Can you work these out from the model? Positions are in its coordinate system, mm. Round coordinates to 2 decimals unless told otherwise and drop trailing zeros. Order: outer loops, then holes, each group sorted by start corner. A loop starts at its lowest first (then second) coordinate and runs counter-clockwise, first axis right, second up. Notation, with made-up numbers: M 6,51 L 25,51 A19 cw 25,58 Z; hole C 40,65.25 d11. An arc over 180 degrees is marked long. One line per question, with ' | ' between items.
```python
from build123d import *

# Parameters (mm, degrees)
F1_DEPTH = 1460
F3_D     = 5.5
F3_DEPTH = 14.4
F3_TIP   = 1.6523667023
F5_DEPTH = 50.001


# Not quite as in the source:
# - a feature names something its author has since deleted; it is built from what else it names


with BuildPart() as f1:
    # F0 (on Front) → F1 (new body)
    with BuildSketch(Plane.XZ):
        with BuildLine():
            Line((-20, -50), (20, -50))
            ThreePointArc((20, -50), (23.5355339059, -48.5355339059), (25, -45))
            Line((25, -45), (25, 45))
            ThreePointArc((25, 45), (23.5355339059, 48.5355339059), (20, 50))
            Line((20, 50), (-20, 50))
            ThreePointArc((-20, 50), (-23.5355339059, 48.5355339059), (-25, 45))
            Line((-25, 45), (-25, -45))
            ThreePointArc((-25, -45), (-23.5355339059, -48.5355339059), (-20, -50))
        make_face()
        with BuildLine():
            ThreePointArc((-17.5, -45), (-19.267766953, -44.267766953), (-20, -42.5))
            Line((-20, -42.5), (-20, 42.5))
            ThreePointArc((-20, 42.5), (-19.267766953, 44.267766953), (-17.5, 45))
            Line((-17.5, 45), (17.5, 45))
            ThreePointArc((17.5, 45), (19.267766953, 44.267766953), (20, 42.5))
            Line((20, 42.5), (20, -42.5))
            ThreePointArc((20, -42.5), (19.267766953, -44.267766953), (17.5, -45))
            Line((17.5, -45), (-17.5, -45))
        make_face(mode=Mode.SUBTRACT)
    extrude(amount=-F1_DEPTH)

    # F3
    with Locations(Plane.XY.offset(50)):
        with Locations((0, 50), (0, 250), (0, 450), (0, 650), (0, 850), (0, 1050), (0, 1250), (0, 1450)):
            Hole(F3_D / 2, depth=F3_DEPTH)
            with Locations((0, 0, -(F3_DEPTH + F3_TIP / 2))):  # 118° drill point
                Cone(0, F3_D / 2, F3_TIP, mode=Mode.SUBTRACT)

    # F4 (on face) → F5 (cut, through all)
    with BuildSketch(Plane.YZ.offset(25)):
        with BuildLine():
            Line((1450.4894832185, 29.8696045958), (1450.4894832185, 35.6303954042))
            ThreePointArc((1450.4894832185, 35.6303954042), (1444.1498086534, 42.4982734143), (1437.5003786468, 35.9298411402))
            Line((1437.5003786468, 35.9298411402), (1437.5003786468, 29.5701588598))
            ThreePointArc((1437.5003786468, 29.5701588598), (1444.1498086534, 23.0017265857), (1450.4894832185, 29.8696045958))
        make_face()
        with BuildLine():
            Line((1437.5008297564, -29.6038563662), (1437.5000000547, -35.999156715))
            ThreePointArc((1437.5000000547, -35.999156715), (1444.0002415297, -42.4999999955), (1450.4999998647, -35.9986736556))
            Line((1450.4999998647, -35.9986736556), (1450.4987003133, -29.6299778371))
            ThreePointArc((1450.4987003133, -29.6299778371), (1444.0130628488, -23.000013126), (1437.5008297564, -29.6038563662))
        make_face()
    extrude(amount=-F5_DEPTH, mode=Mode.SUBTRACT)


solid = f1.part
```
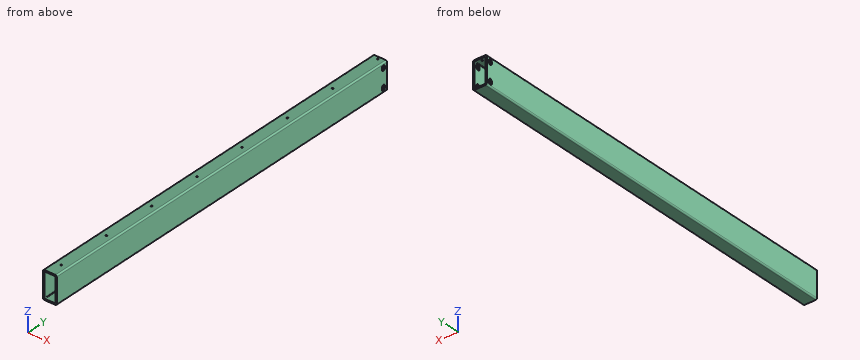
(1) Please list where these lines run through material, in increasing order: probe 1 along Z at (x, y) = (-14.5, 572); probe 2 along X at (y, z) = (526, -38); probe 3 along Z at (x, y) = (18.5, 610.5). Write a range as [from, to].
Final values:
probe 1: [-50, -45], [45, 50] | probe 2: [-25, -20], [20, 25] | probe 3: [-50, -44.79], [44.79, 50]
(2) If we section it at A-A on z = -6: Please give me the cut outline in (x, y), plus the area to 3 significant figures.
Final values:
outline: M -25,0 L -20,0 L -20,1460 L -25,1460 Z; M 20,0 L 25,0 L 25,1460 L 20,1460 Z | area: 14,600 mm^2
(3) If we section it at B-B on y = 1032.5: Please give me the cut outline in (x, z).
Final values:
outline: M -25,-45 A5 ccw -20,-50 L 20,-50 A5 ccw 25,-45 L 25,45 A5 ccw 20,50 L -20,50 A5 ccw -25,45 Z; hole M -20,-42.5 A2.5 ccw -17.5,-45 L 17.5,-45 A2.5 ccw 20,-42.5 L 20,42.5 A2.5 ccw 17.5,45 L -17.5,45 A2.5 ccw -20,42.5 Z
(4) Will these pins go through, and if not, where does the flat tip stop? pin 1 Ø3.5 at (x, y) = (0, 1250) entering from +Z; pin 2 Ø1.5 at (x, z) = (-23.5, -32.5) entering from -Y.
Final values:
pin 1: z = -45 | pin 2: y = 0
